Autodesk Inventor part; units mm, degrees
ref_plane "YZ Plane" through (0, 0, 0) normal (1, 0, 0) x (0, 1, 0)
ref_plane "XZ Plane" through (0, 0, 0) normal (0, 1, 0) x (-1, 0, 0)
ref_plane "XY Plane" through (0, 0, 0) normal (0, 0, 1) x (1, 0, 0)
sketch "Sketch1" plane through (0, 0, 0) normal (0, 1, 0) x (-1, 0, 0)
  line L0 (20, -0.25) -> (20, 20)
  line L1 (20, 20) -> (-20.5, 20)
  line L2 (-20.5, 20) -> (-20.5, -0.25)
  line L3 (20, 9.875) -> (-20.5, 9.875)
  dimension "d49" = 40.5
extrude "Extrusion1" add sketch "Sketch1" along normal mid plane 40
sketch "Sketch6" plane through (0, 0, 0) normal (0, 0, 1) x (1, 0, 0)
  line L0 (0, 0) -> (-15, 0)
  line L1 (-15, 0) -> (-15, -15)
  line L2 (-15, -15) -> (15, -15)
  line L3 (15, -15) -> (15, 15)
  line L4 (15, 15) -> (-15, 15)
  line L5 (-15, 15) -> (-15, 0)
  dimension "d64" = 15
  dimension "d65" = 15
  dimension "d66" = 90
  dimension "d67" = 30
  dimension "d68" = 90
  dimension "d69" = 30
  dimension "d70" = 90
  dimension "d71" = 30
  dimension "d72" = 90
extrude "Extrusion6" add sketch "Sketch6" along normal blind 40.4
hole "Hole2" at (0, 0, 40.4) direction (0, 0, -1) diameter 19 depth 15
fillet "Fillet3" [suppressed]
sketch "Sketch8" plane through (0, 0, 0) normal (0, 0, -1) x (-1, 0, 0)
  line L0 (15, -15) -> (-15, -15)
  line L1 (-15, -15) -> (-15, 15)
  line L2 (-15, 15) -> (15, 15)
  line L3 (15, 15) -> (15, -15)
  point P0 (0, 0)
extrude "Extrusion8" cut sketch "Sketch8" against normal blind 10
sketch "Sketch10" plane through (-20, 20, 20) normal (0, 0, 1) x (1, 0, 0)
  line L0 (0, 0) -> (-6, 0)
  line L1 (-6, 0) -> (-6, -40)
  line L2 (-6, -40) -> (0, -40)
  line L3 (0, -40) -> (0, 0)
  line L4 (40.5, 0) -> (46.5, 0)
  line L5 (46.5, 0) -> (46.5, -40)
  line L6 (46.5, -40) -> (40.5, -40)
  line L7 (40.5, -40) -> (40.5, 0)
  point P0 (20, -20)
  dimension "d73" = 6
  dimension "d74" = 6
  dimension "d75" = 40.5
extrude "Extrusion9" add sketch "Sketch10" against normal blind 29
hole "Hole3" at (23.5, 14, -9) direction (0, 0, 1) diameter 3.242 depth 11.8 tip angle 118
hole "Hole4" at (23.5, -14, -9) direction (0, 0, 1) diameter 3.242 depth 11.8 tip angle 118
hole "Hole5" at (-23, 14, -9) direction (0, 0, 1) diameter 3.242 depth 11.8 tip angle 118
hole "Hole6" at (-23, -14, -9) direction (0, 0, 1) diameter 3.242 depth 11.8 tip angle 118
properties part number "suporte-barra" material "Steel, Carbon"
Read the model definition and answer for the solid it produces. Units are mm, in the model's axes. A direction names the side the tool comes from. Round coordinates to 2 decimals unless told otherwise and drop trailing zeros. Loops run counter-clockwise (first coordinate to the right, second up) from the corner with the lowest first, then second, coordinate; pieces in that order, holes last.
Q1. Which of the six approach directions +Z, -Z, +X, -X, +Y, -Y give full straight-line access (tool end or side, diameter ignored) to faces 5 (the face through (0, 17, 9.875)), 6 (the face through (24.121, -12.503, -3.017)), 7 (the face through (0, -15, 30))?
Q2. Determine the mould class of faces 1 (the face through (1, -20, 12)), 2 (the face through (23.225, 13.939, 3.605)), 3 (the face through (-20, 0, 1)), 4 (the face through (-26, 0, 6)) for opening direction X: released by +X, released by -X, zero draft, split by the parting line, or undercut.
Q3. Section A-A on z = 1.5 is taken. Write down the section's boundary in (x, y), and give its area (3 significant figures).
Q4. Section B-B on z = 7.5 is taken. Write down the section's boundary in (x, y).
Q5. Consider probe 1 along X at (y, z) = (-14, -4.5); probe 2 along Y at (x, z) = (-23, -5.75); probe 3 along X at (y, z) = (0, 30.75). Determine where each line is inside the solid, lowest interval first.
Q6. Section C-C on x = 0 is taken. Write down the section's boundary in (y, z) (3 decimals), and give its area (3 significant figures).
Q7. Each of these flat-tipped pins is pushed along its axis until it touches: pin 1 (3 mm diameter, centred on x = 9, z = 27.5, fed in from -Y); pin 2 (1.9 mm diameter, centred on x = 23.5, y = 14, fed in from +Z); pin 3 (3 mm diameter, centred on x = -23, y = 14, fed in from -Z). Where does it stop, or does it pass through?
Q8. Section D-D on y = 11 is taken. Write down the section's boundary in (x, z) (3 decimals), and give its area (3 significant figures).
Output:
1. face 5: -Z, +Y, -Y
1. face 6: -Z
1. face 7: +Z, +X, -X, -Y
2. face 1: zero draft
2. face 2: undercut
2. face 3: undercut
2. face 4: released by -X
3. outline: (-26, -20) - (-20, -20) - (-20, 20) - (-26, 20) - close; (20.5, -20) - (26.5, -20) - (26.5, 20) - (20.5, 20) - close; hole circle Ø3.24 at (-23, -14); hole circle Ø3.24 at (-23, 14); hole circle Ø3.24 at (23.5, -14); hole circle Ø3.24 at (23.5, 14)
3. area: 447 mm2
4. outline: (-26, -20) - (-20, -20) - (-20, 20) - (-26, 20) - close; (20.5, -20) - (26.5, -20) - (26.5, 20) - (20.5, 20) - close
5. probe 1: x = -26 to -24.62, -21.38 to -20, 20.5 to 21.88, 25.12 to 26.5
5. probe 2: y = -20 to -15.62, -12.38 to 12.38, 15.62 to 20
5. probe 3: x = -15 to -9.5, 9.5 to 15
6. outline: (-20, 9.875) - (-15, 9.875) - (-15, 10) - (15, 10) - (15, 9.875) - (20, 9.875) - (20, 20) - (15, 20) - (15, 40.4) - (9.5, 40.4) - (9.5, 25.4) - (-9.5, 25.4) - (-9.5, 40.4) - (-15, 40.4) - (-15, 20) - (-20, 20) - close
6. area: 728 mm2
7. pin 1: stops at y = -15
7. pin 2: stops at z = 20
7. pin 3: stops at z = 2.87
8. outline: (-26, -9) - (-20, -9) - (-20, 9.875) - (-15, 9.875) - (-15, 10) - (15, 10) - (15, 9.875) - (20.5, 9.875) - (20.5, -9) - (26.5, -9) - (26.5, 20) - (15, 20) - (15, 40.4) - (-15, 40.4) - (-15, 20) - (-26, 20) - close
8. area: 1,370 mm2
